Geometry: final body of the model. Coordinates: model frame, mm. Face numbers are marked on the shaded views. A direction names the side the tool comes from. Coordinates: 2 decimals unless noted, no trailing zeros. Order: outer loops, then holes, each group sorted by start corner. A loop starts at its lowest first (then second) coordinate and runs counter-clockwise, first axis right, second up. Notation, with made-up numbers: (7, 19) -> (61, 19) arc R27 ccw to (61, 57) -> close; hole circle Ø10 at (3, 5.5). An arc over 180 degrees is marked (long way). Answer in a Markdown table with one row per item. Add a question column.
1) Ray query, line 1 (Z direction, x = 24.25, y = 4.25); line 2 (Y direction, x = 4.25, z = -6.5). Return the intervals inside material, ascending. Write a range as from..to.
2) Section query A-A on y = 5. Return the cut outline in (x, z), then the cut area to 3 significant figures.
3) Section query C-C on z = -15.5. Return the cut outline in (x, y), then the cut area to 3 significant figures.
4) Pull-direction query (Z, two-part tool) for the marked faces 1, 2 and 3; classes: +Z half, -Z half, draft (parallel to the pull), parting line (faces both ways), or undercut.
5) Set-up query: the marked faces 4 and 5. Return all of +Z, -Z, +X, -X, +Y, -Y with unobstructed straight access to the full face (end or side cutting, diameter ignored); none if empty.
6) Section query B-B on x = 21.5. Return the cut outline in (y, z), then the cut area to 3 significant figures.
7) Contact query for flat-ended pins moving along their axis: P1, Ø6.5, axis at x = 12, z = -15, coming from the -Y side; P2, Ø1.5, axis at y = 4.5, z = -16, coming from the -X side. Output: stop coordinate, or through.
```python
from build123d import *

# Parameters (mm, degrees)
F1_DEPTH = 25.4


with BuildPart() as f1:
    # F0 (on Right) → F1 (new body)
    with BuildSketch(Plane.YZ):
        Polygon((25.4, 0), (0, 0), (0, -2.695372), (0, -6.35), (6.35, -6.35), (6.35, -19.05), (0, -19.05), (0, -25.4), (25.4, -25.4), align=None)
    extrude(amount=F1_DEPTH)


solid = f1.part
```
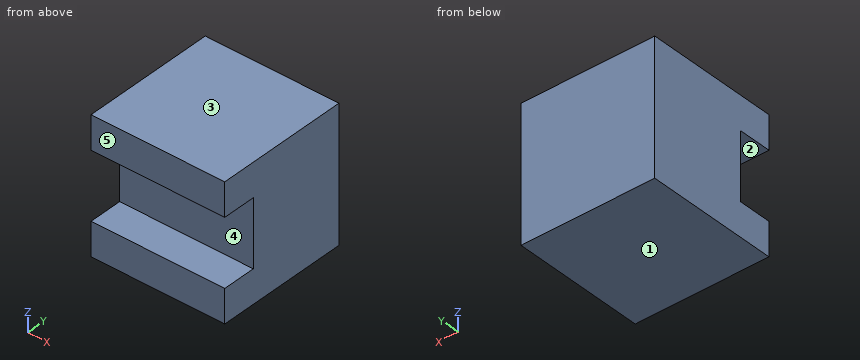
Result:
| question | item | result |
|---|---|---|
| 1 | line 1 | -25.4..-19.05, -6.35..0 |
| 1 | line 2 | 6.35..25.4 |
| 2 | outline | (0, -25.4) -> (25.4, -25.4) -> (25.4, -19.05) -> (0, -19.05) -> close; (0, -6.35) -> (25.4, -6.35) -> (25.4, 0) -> (0, 0) -> close |
| 2 | area | 323 mm2 |
| 3 | outline | (0, 6.35) -> (25.4, 6.35) -> (25.4, 25.4) -> (0, 25.4) -> close |
| 3 | area | 484 mm2 |
| 4 | face 1 | -Z half |
| 4 | face 2 | undercut |
| 4 | face 3 | +Z half |
| 5 | face 4 | +X, -X, -Y |
| 5 | face 5 | +Z, -Z, +X, -X, -Y |
| 6 | outline | (0, -25.4) -> (25.4, -25.4) -> (25.4, 0) -> (0, 0) -> (0, -6.35) -> (6.35, -6.35) -> (6.35, -19.05) -> (0, -19.05) -> close |
| 6 | area | 565 mm2 |
| 7 | P1 | y = 6.35 |
| 7 | P2 | through |
